Geometry check sheet. Reference: the model listing, model coordinates, mm. A direction names the side the tool comes from. Give positions to 0.01 mm unless a question says otherwise; leave off trailing zeros. Write each loop counter-clockwise with the first axis right and the second up, starting at its lowest first coordinate (ties: lowest second). Pieces come first, ordered by that corner, then holes.
(1) Tool access check on faces 1 (the cylindrical face through (-4.59, 2.95, -4.3)), 2 (the flat face through (-1.5, -7, -6)), 3 (the flat face through (1.5, -7, -6)). Record the directions out of +Z, -Z, +X, -X, +Y, -Y that give a thin tool (end or side, any length) a straight path to the whole face; none if there is none.
(2) Cross-section at D-D (x = -4.5). Record the boundary of the cut face in (y, z).
(3) Mould release check, pull along Y, two halves, no side actions. Record for faces 4 (the flat face through (0, -7.9, -6)), 5 (the cylindrical face through (-1.43, 2.75, -7.4)), 6 (the cylindrical face through (-4.57, -7.167, -13.226)): +Y half, -Y half, draft (parallel to the pull), parting line (faces both ways), or undercut.
(4) Thickness scan on line 1 along Y through (x, z) = (0, -4.25); line 2 along Z through (x, y) = (-4.2, 0); line 3 along X through (y, z) = (0, -9.25). Record the ranges inside material, lowest first.
(5) Depth check by flat-ended pin: P1, Ø1.5, axis at y = 1, z = -13, coming from the -X side; P2, Ø3.5, axis at x = -0.5, z = -3, coming from the -Y side; P3, Ø8, axis at y = 5.5, z = -1.5, coming from the +X side. Enter the tip coordinate at first touch or a pass-through.
(6) Cross-section at B-B (y = -2). Record the boundary of the cut face in (x, z), and give its area (3 significant figures).
(7) Cross-section at C-C (z = -4). Record the boundary of the cut face in (x, y).
(8) Cross-section at A-A (x = 0). Record the boundary of the cut face in (y, z), and give its area (3 significant figures).
Autodesk Inventor part; units mm, degrees
ref_plane "Work Plane1" through (-6.4, 0, 0) normal (-1, 0, 0) x (0, -1, 0)
ref_plane "YZ Plane" through (0, 0, 0) normal (1, 0, 0) x (0, 1, 0)
ref_plane "XZ Plane" through (0, 0, 0) normal (0, 1, 0) x (-1, 0, 0)
sketch "Sketch1" plane through (0, 0, 0) normal (0, 1, 0) x (-1, 0, 0)
  line L0 (0, 0) -> (0, -7)
  circle A0 centre (0, -7) radius 1.55
  line L1 (3.1, 0) -> (6.4, 0)
  circle A1 centre (0, -7) radius 4
  line L2 (0, -11) -> (0, -15)
  line L3 (3.1, -15) -> (3.1, 0)
  line L4 (6.4, 0) -> (6.4, -11.5)
  line L5 (6.35, -15) -> (3.1, -15)
  line L6 (3.1, -15) -> (8.5, -15)
  line L7 (8.5, -15) -> (8.5, -11.5)
  line L8 (8.5, -11.5) -> (6.4, -11.5)
  line L9 (6.4, 0) -> (7.9, 0)
  line L10 (7.9, 0) -> (7.9, -11.5)
  line L11 (6.4, 0) -> (4.9, 0)
  line L12 (4.9, 0) -> (4.9, -11.5)
  line L13 (4.9, -11.5) -> (6.4, -11.5)
  dimension "d4" = 8
  dimension "d0" = 7
  dimension "d1" = 3.1
  dimension "d2" = 6.4
  dimension "d3" = 3.1
  dimension "d5" = 4
  dimension "d6" = 8.5
  dimension "d7" = 3.5
  dimension "d18" = 1.5
  dimension "d19" = 1.5
revolve "Revolution1" add sketch "Sketch1" angle 360 about axis through (0, 0, 0) along (0, 0, -1) picked at (3.2637, -7.5872) contours L3 L1 L12 L13 L8 L7 L6 L5 A1 | A1 L3 | L1 L4 L13 L12
ref_plane "Work Plane1" through (-6.4, 0, 0) normal (-1, 0, 0) x (0, -1, 0)
sketch "Sketch2" plane through (-6.4, 0, 0) normal (-1, 0, 0) x (0, -1, 0)
  line L0 (0, 0) -> (0, -7)
  circle A0 centre (0, -7) radius 1.55
  circle A1 centre (0, -7) radius 4
  dimension "d11" = 7
  dimension "d12" = 3.1
  dimension "d13" = 8
extrude "Extrusion2" cut sketch "Sketch2" against normal blind 30 contours A0
extrude "Extrusion3" cut sketch "Sketch2" against normal blind 3
sketch "Sketch3" plane through (0, 0, 0) normal (0, 0, 1) x (1, 0, 0)
  circle A0 centre (0, 0) radius 3.1
  line L0 (0, -3.1) -> (0, -6.4)
  circle A1 centre (0, 0) radius 6.4
  line L1 (0, -6.4) -> (0, -7.9)
  line L2 (0, -6.4) -> (0, -4.9)
  line L3 (0, -4.9) -> (-1.5, -4.9)
  line L4 (-1.5, -4.9) -> (-1.5, -7.9)
  line L5 (-1.5, -7.9) -> (0, -7.9)
  line L6 (0, -7.9) -> (1.5, -7.9)
  line L7 (1.5, -7.9) -> (1.5, -4.9)
  line L8 (1.5, -4.9) -> (0, -4.9)
  dimension "d20" = 1.5
  dimension "d21" = 1.5
  dimension "d22" = 1.5
  dimension "d23" = 1.5
extrude "Extrusion4" add sketch "Sketch3" against normal blind 11.5 contours L8 L7 A1 L0 | L0 A1 L4 L3 | L1 L5 L4 A1 | A1 L7 L6 L1
properties part number "dc_to_omni_coupler_small"
Reply:
1. face 1: -X
1. face 2: +Z, -X, -Y
1. face 3: +Z, +X, -Y
2. outline: (-7.21, -15) - (7.21, -15) - (7.21, -11.5) - (4.55, -11.5) - (4.55, 0) - (-4.55, 0) - (-4.55, -11.5) - (-7.21, -11.5) - close; hole circle Ø8 at (0, -7)
3. face 4: -Y half
3. face 5: undercut
3. face 6: parting line
4. line 1: y = -7.9 to -3.1, 3.1 to 6.4
4. line 2: z = -15 to -11, -3 to 0
4. line 3: x = -3.4 to -3.1, 3.1 to 6.4
5. P1: stops at x = -8.5
5. P2: stops at y = -7.9
5. P3: stops at x = 6.22
6. outline: (-8.26, -15) - (-2.37, -15) - (-2.37, 0) - (-6.08, 0) - (-6.08, -3.54) - (-3.4, -3.54) - (-3.4, -10.46) - (-6.08, -10.46) - (-6.08, -11.5) - (-8.26, -11.5) - close; (2.37, -15) - (8.26, -15) - (8.26, -11.5) - (6.08, -11.5) - (6.08, 0) - (2.37, 0) - close
6. area: 108 mm2
7. outline: (-5.83, -2.65) arc R6.4 ccw to (-1.5, -6.22) - (-1.5, -7.9) - (1.5, -7.9) - (1.5, -6.22) arc R6.4 ccw (long way) to (-5.83, 2.65) - (-3.4, 2.65) - (-3.4, -2.65) - close; hole circle Ø6.2 at (0, 0)
8. outline: (-8.5, -15) - (-3.1, -15) - (-3.1, 0) - (-7.9, 0) - (-7.9, -11.5) - (-8.5, -11.5) - close; (3.1, -15) - (8.5, -15) - (8.5, -11.5) - (6.4, -11.5) - (6.4, 0) - (3.1, 0) - close
8. area: 131 mm2
